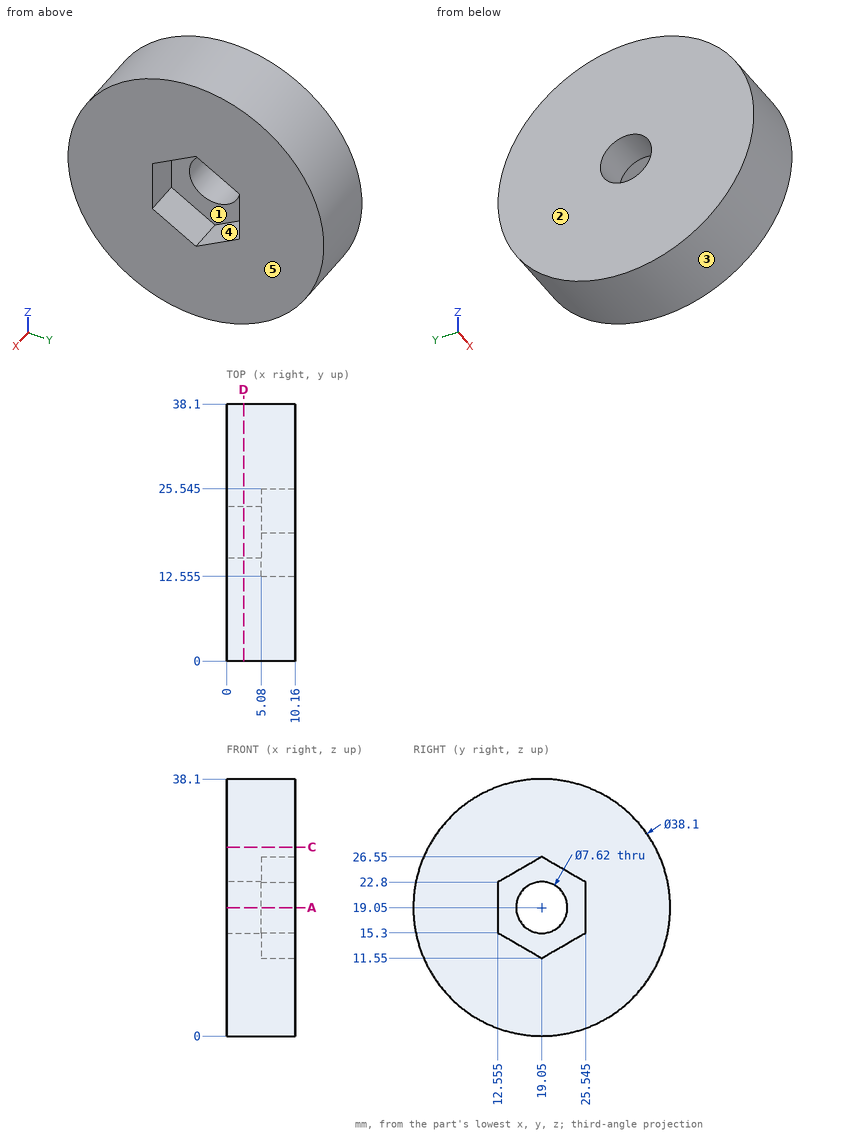
Can you work these out from the drawing? Everything is in mm from the part's minimum corner. A direction names the side the tool comes from. Give positions to 0.01 mm unless a question says otherwise; leave off trailing zeros. Order: outer loops, then holes, each group sorted by start corner. A loop starts at its lowest first (then second) coordinate and runs counter-clockwise, first axis right, second up. Notation, with made-up numbers: M -16,62 L 14,62 A26 cw 14,98 Z; hole C 17.25,-15.5 d11. An arc over 180 degrees is marked long. One line per question, with ' | ' between items.
1. I'm going to push flat-ended pins straight in: pin 1 (5 mm diameter, centred on x = 7, y = 15.5, fed in from +Z); pin 2 (1.5 mm diameter, centred on x = 5.5, y = 27, fed in from -Z); pin 3 (6 mm diameter, centred on x = 1.5, z = 11, fed in from +Y). Where does each tip first touch, or does it pass through?
Results:
pin 1: z = 38.07 | pin 2: z = 1.41 | pin 3: y = 37.42
2. I want a section at C-C (z = 28). List the corners of the cut face in (x, y) for me.
Results:
outline: M 0,2.23 L 10.16,2.23 L 10.16,35.87 L 0,35.87 Z
3. I want a section at A-A (z = 19.05). List the corners of the cut face in (x, y) for me (1 decimal), and give its area (3 significant figures).
Results:
outline: M 0,0 L 10.2,0 L 10.2,12.6 L 5.1,12.6 L 5.1,15.2 L 0,15.2 Z; M 0,22.9 L 5.1,22.9 L 5.1,25.5 L 10.2,25.5 L 10.2,38.1 L 0,38.1 Z | area: 282 mm²
4. If I drill on line 1 (Y direction, x = 1.1, z = 19.05); line 2 (Y direction, x = 4.5, z = 19.5) (1 decimal); line 3 (Z direction, x = 7.75, y = 24.5), over which ranges is the centre line in solid material (lowest first)?
Results:
line 1: 0 to 15.24, 22.86 to 38.1 | line 2: 0 to 15.3, 22.8 to 38.1 | line 3: 0.8 to 14.7, 23.4 to 37.3
5. I want a section at D-D (x = 2.5). List the corners of the cut face in (y, z) for me.
Results:
outline: C 19.05,19.05 d38.1; hole C 19.05,19.05 d7.62
6. We'd pull the mould along Z, two halves only. Please class the marked faces 3, 4 and 5: +Z half, -Z half, draft (parallel to the pull), parting line (faces both ways), or undercut.
Results:
face 3: parting line | face 4: undercut | face 5: draft
7. For the marked faces 1 and 2, which set-ups out of +Z, -Z, +X, -X, +Y, -Y let a thin tool reach every point of the face, with its end or its side?
Results:
face 1: +X | face 2: +Z, -Z, -X, +Y, -Y
